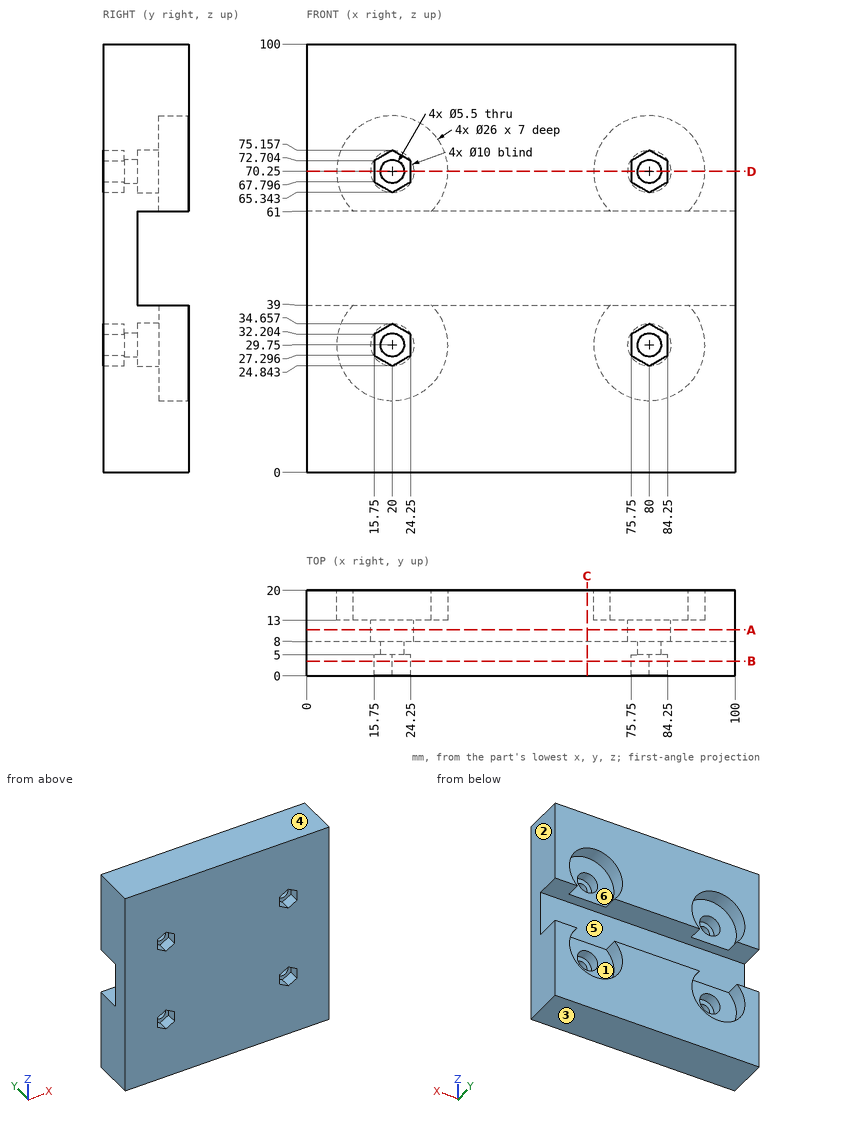
Answer from the drawing. Dimensions are ordinates in mm from the lowest x, y and z of the part. A direction names the side the tool comes from. Give positions to 0.01 mm unless a question says otherwise; leave off trailing zeros. Write each loop counter-clockwise with the first axis right and the second up, starting at its lowest first coordinate (ties: lowest second). Pieces come first, ordered by that corner, then holes.
1) Section A-A (y = 10.75) is taken. Write down the section's boundary in (x, z), and give its area (3 significant figures).
2) Given P1, Ø7, axis at x = 80, z = 29.75, coming from the +Y side; P2, Ø2.5, axis at x = 80.5, z = 31, coming from the -Y side; P3, Ø18, axis at x = 80.5, z = 33, coming from the +Y side, each flat-ended and moving along its own axis, determine where each tip first touches the part or whether it passes through.
3) For a pull along Z with two mould halves and no side action, classify the marked faces 1, 2 and 3 as pulls with the +Z half, pulls with the -Z half, needs draft (parallel to the pull), parting line crosses it, or undercut.
4) Section C-C (x = 65.5) is taken. Write down the section's boundary in (y, z), and give its area (3 significant figures).
5) Find the intervals of material crossed by L1, parallel to X at y = 6.5, z = 70.25; L2, parallel to X at y = 2, z = 28.5; L3, parallel to Z at x = 67.5, y = 12.25, in increasing order.
6) Section D-D (z = 70.25) is taken. Count the separate pieces of the cut face and the enclosed holes in it, and give its area (3 significant figures).
7) Section B-B (y = 3.5) is taken. Write down the section's boundary in (x, z), and give its area (3 significant figures).
8) A tool of negligible diameter and unlimited length cuts with its end or side. For the marked faces 4, 5 and 6, from which of +Z, -Z, +X, -X, +Y, -Y can it reach the whole face along a straight path? Write none if from no direction.
Response:
1. outline: (0, 0) - (100, 0) - (100, 39) - (0, 39) - close; (0, 61) - (100, 61) - (100, 100) - (0, 100) - close; hole circle Ø10 at (20, 29.75); hole circle Ø10 at (20, 70.25); hole circle Ø10 at (80, 29.75); hole circle Ø10 at (80, 70.25)
1. area: 7,490 mm2
2. P1: stops at y = 8
2. P2: passes through
2. P3: stops at y = 13
3. face 1: undercut
3. face 2: needs draft
3. face 3: pulls with the -Z half
4. outline: (0, 0) - (20, 0) - (20, 39) - (8, 39) - (8, 61) - (20, 61) - (20, 100) - (0, 100) - close
4. area: 1,740 mm2
5. L1: x = 0 to 17.25, 22.75 to 77.25, 82.75 to 100
5. L2: x = 0 to 15.75, 24.25 to 75.75, 84.25 to 100
5. L3: z = 0 to 39, 61 to 100
6. separate pieces: 3
6. enclosed holes: 0
6. area: 1,420 mm2
7. outline: (0, 0) - (100, 0) - (100, 100) - (0, 100) - close; hole (15.75, 27.3) - (20, 24.84) - (24.25, 27.3) - (24.25, 32.2) - (20, 34.66) - (15.75, 32.2) - close; hole (15.75, 67.8) - (20, 65.34) - (24.25, 67.8) - (24.25, 72.7) - (20, 75.16) - (15.75, 72.7) - close; hole (75.75, 27.3) - (80, 24.84) - (84.25, 27.3) - (84.25, 32.2) - (80, 34.66) - (75.75, 32.2) - close; hole (75.75, 67.8) - (80, 65.34) - (84.25, 67.8) - (84.25, 72.7) - (80, 75.16) - (75.75, 72.7) - close
7. area: 9,750 mm2
8. face 4: +Z, +X, -X, +Y, -Y
8. face 5: +X, -X, +Y
8. face 6: +Y
